Here's how the part is built. I have some questions about the finished solid (model axes, mm). A direction names the side the tool comes from. Round coordinates to 2 decimals unless told otherwise and drop trailing zeros. Loops run counter-clockwise (first coordinate to the right, second up) from the corner with the lowest first, then second, coordinate; pieces in that order, holes last. Notation, with made-up numbers: (44, 52) -> (79, 52) arc R14 cw to (79, 68) -> close; hole circle Ø3 at (43, 56.25). An arc over 180 degrees is marked (long way). One line per item, written item: value. Start each with the question number.
```python
from build123d import *

# Parameters (mm, degrees)
MICRO_SERVO_MOUNT_BASE_PART_CAMERA_TUR_DEPTH = 17.2796
MICRO_START                                  = -8.24
MICRO_SERVO_MOUNT_BASE_PART_CAMERA_3_O_R     = 1.2
MICRO_SERVO_MOUNT_BASE_PART_CAMERA_3_DEPTH   = 16.48
SKETCH7_W                                    = 46
SKETCH7_H                                    = 30
BOSS_EXTRUDE1_DEPTH                          = 3.5
BOSS_EXTRUDE1_DIRECTION_2_REACH              = 35.842
M2_5_CLEARANCE_HOLE1_D                       = 2.9
FILLET1_R                                    = 3
BOSS_EXTRUDE2_DEPTH                          = 10
SKETCH11_R                                   = 2.5
BOSS_EXTRUDE3_DEPTH                          = 8
SKETCH14_W                                   = 17.2796
SKETCH14_H                                   = 27.0711
BOSS_EXTRUDE5_DEPTH                          = 1
BOSS_EXTRUDE4_DEPTH                          = 5
SKETCH13_W                                   = 1.5
SKETCH13_H                                   = 4.25
CUT_EXTRUDE1_DEPTH                           = 39.791353434
FILLET2_R                                    = 2
CUT_EXTRUDE2_DEPTH                           = 2.25
CUT_EXTRUDE3_DEPTH                           = 61.415771958
CHAMFER1_SIZE                                = 0.5


with BuildPart() as part:
    # Micro Servo Mount Base Part - Camera Tur: read off the stored shape, not the designer's step
    # Micro Servo Mount Base Part - Camera 2 → Micro Servo Mount Base Part - Camera Tur (new body)
    with BuildSketch(Plane.YZ):
        Polygon((-23.9811, 0.5), (-16.8311, 0.5), (-16.8311, 6.24), (6.24, 6.24), (6.24, 2.4478), (8.74, 2.4478), (8.74, -2.4478), (6.24, -2.4478), (6.24, -6.24), (-16.8311, -6.24), (-16.8311, -0.5), (-23.9811, -0.5), (-23.9811, -2), (-18.8311, -2), (-18.8311, -8.24), (8.24, -8.24), (8.24, -5), (10.24, -3.5), (10.24, 3.5), (8.24, 5), (8.24, 8.24), (-18.8311, 8.24), (-18.8311, 2), (-23.9811, 2), align=None)
    extrude(amount=MICRO_SERVO_MOUNT_BASE_PART_CAMERA_TUR_DEPTH)

    # Micro Servo Mount Base Part - Camera 3 o → Micro Servo Mount Base Part - Camera 3 (cut)
    with BuildSketch(Plane.XY.offset(MICRO_START)):
        with BuildLine():
            Line((0, -23.9811), (3, -23.9811))
            ThreePointArc((3, -23.9811), (0.878679656, -23.102420344), (0, -20.9811))
            Line((0, -20.9811), (0, -23.9811))
        make_face()
        with BuildLine():
            ThreePointArc((17.2796, -20.9811), (16.400920344, -23.102420344), (14.2796, -23.9811))
            Line((14.2796, -23.9811), (17.2796, -23.9811))
            Line((17.2796, -23.9811), (17.2796, -20.9811))
        make_face()
        with Locations((3, -20.9811)):
            Circle(MICRO_SERVO_MOUNT_BASE_PART_CAMERA_3_O_R)
        with Locations((14.2796, -20.9811)):
            Circle(MICRO_SERVO_MOUNT_BASE_PART_CAMERA_3_O_R)
    extrude(amount=MICRO_SERVO_MOUNT_BASE_PART_CAMERA_3_DEPTH, mode=Mode.SUBTRACT)

    # Sketch7 → Boss-Extrude1 (add)
    with BuildSketch(Plane.XY.offset(8.24)):
        with Locations((13.6398, 0)):
            Rectangle(SKETCH7_W, SKETCH7_H)
    extrude(amount=BOSS_EXTRUDE1_DEPTH)

    # Boss-Extrude1 direction 2: up to this face of the body (flat: up to its plane)
    boss_extrude1_direction_2_end = Plane(part.part.faces().sort_by_distance((8.6398, -5.29555, 6.24))[0])
    # Sketch7 → Boss-Extrude1 direction 2 (add, up to the picked face)
    with BuildSketch(Plane.XY.offset(8.24), mode=Mode.PRIVATE) as boss_extrude1_direction_2_sk1:
        with Locations((13.6398, 0)):
            Rectangle(SKETCH7_W, SKETCH7_H)
    boss_extrude1_direction_2_tool1 = split(extrude(boss_extrude1_direction_2_sk1.sketch, amount=-BOSS_EXTRUDE1_DIRECTION_2_REACH, mode=Mode.PRIVATE), bisect_by=boss_extrude1_direction_2_end, keep=Keep.BOTH, mode=Mode.PRIVATE)
    add(boss_extrude1_direction_2_tool1.solids().sort_by(Axis((13.6398, 0, 8.24), (0, 0, -1)))[0])

    # M2.5 Clearance Hole1 (through all)
    with Locations(Plane.XY.offset(11.74)):
        with Locations((-6.3602, 12), (33.6398, 12), (33.6398, -12), (-6.3602, -12)):
            Hole(M2_5_CLEARANCE_HOLE1_D / 2)

    # Fillet1
    fillet1_edges = [part.edges().sort_by_distance(p)[0] for p in [
        (36.6398, -15, 8.99),
        (-9.3602, 15, 8.99),
        (-9.3602, -15, 8.99),
        (36.6398, 15, 8.99),
    ]]
    fillet(fillet1_edges, radius=FILLET1_R)

    # Sketch10 → Boss-Extrude2 (add)
    with BuildSketch(Plane(origin=(36.6398, 0, 0), x_dir=(0, 0, -1), z_dir=(1, 0, 0))):
        with BuildLine():
            Line((-6.24, 3.5), (0, 3.5))
            ThreePointArc((0, 3.5), (3.5, 0), (0, -3.5))
            Line((0, -3.5), (-6.24, -3.5))
            Line((-6.24, -3.5), (-6.24, 3.5))
        make_face()
    extrude(amount=-BOSS_EXTRUDE2_DEPTH)

    # Sketch11 → Boss-Extrude3 (add)
    with BuildSketch(Plane(origin=(36.6398, 0, 0), x_dir=(0, 0, -1), z_dir=(1, 0, 0))):
        Circle(SKETCH11_R)
    extrude(amount=BOSS_EXTRUDE3_DEPTH)

    # Sketch14 → Boss-Extrude5 (add)
    with BuildSketch(Plane(origin=(0, 0, -8.24), x_dir=(-1, 0, 0), z_dir=(0, 0, -1))):
        with Locations((-8.6398, -5.29555)):
            Rectangle(SKETCH14_W, SKETCH14_H)
    extrude(amount=BOSS_EXTRUDE5_DEPTH)

    # Sketch12 → Boss-Extrude4 (add, symmetric)
    with BuildSketch(Plane(origin=(0, -6.87055, 0), x_dir=(1, 0, 0), z_dir=(0, 1, 0))):
        Polygon((0, 9.74), (0.5148, 9.74), (0.5148, 9.24), (0, 9.24), (0, 6.24), (-1.5, 6.24), (-1.5, 9.74), align=None)
        Polygon((17.2796, 6.24), (18.7796, 6.24), (18.7796, 9.74), (17.2796, 9.74), (16.7648, 9.74), (16.7648, 9.24), (17.2796, 9.24), align=None)
    extrude(amount=BOSS_EXTRUDE4_DEPTH, both=True)

    # Sketch13 → Cut-Extrude1 (cut, through all)
    with BuildSketch(Plane(origin=(18.7796, 0, 0), x_dir=(0, 0, -1), z_dir=(1, 0, 0))):
        with Locations((6.99, -6.87055)):
            Rectangle(SKETCH13_W, SKETCH13_H)
    extrude(amount=-CUT_EXTRUDE1_DEPTH, mode=Mode.SUBTRACT)

    # Fillet2
    fillet2_edges = [part.edges().sort_by_distance(p)[0] for p in [
        (8.6398, -18.8311, -9.24),
        (8.6398, 8.24, -9.24),
    ]]
    fillet(fillet2_edges, radius=FILLET2_R)

    # Sketch15 → Cut-Extrude2 (cut)
    with BuildSketch(Plane(origin=(0, 0, 6.24), x_dir=(-1, 0, 0), z_dir=(0, 0, -1))):
        Polygon((9.3602, 13.732050808), (6.3602, 15.464101615), (3.3602, 13.732050808), (3.3602, 10.267949192), (6.3602, 8.535898385), (9.3602, 10.267949192), align=None)
        Polygon((9.3602, -10.267949192), (6.3602, -8.535898385), (3.3602, -10.267949192), (3.3602, -13.732050808), (6.3602, -15.464101615), (9.3602, -13.732050808), align=None)
        Polygon((-36.6398, -10.267949192), (-36.6398, -13.732050808), (-33.6398, -15.464101615), (-30.6398, -13.732050808), (-30.6398, -10.267949192), (-33.6398, -8.535898385), align=None)
        Polygon((-36.6398, 13.732050808), (-36.6398, 10.267949192), (-33.6398, 8.535898385), (-30.6398, 10.267949192), (-30.6398, 13.732050808), (-33.6398, 15.464101615), align=None)
    extrude(amount=-CUT_EXTRUDE2_DEPTH, mode=Mode.SUBTRACT)

    # Sketch16 → Cut-Extrude3 (cut, through all)
    with BuildSketch(Plane(origin=(0, 15, 0), x_dir=(1, 0, 0), z_dir=(0, 1, 0))):
        Polygon((2.6398, -11.74), (6.1398, -8.24), (21.1398, -8.24), (24.6398, -11.74), align=None)
    extrude(amount=-CUT_EXTRUDE3_DEPTH, mode=Mode.SUBTRACT)

    # Chamfer1
    chamfer1_edges = [part.edges().sort_by_distance(p)[0] for p in [
        (35.1398, 9.401923789, 6.24),
        (32.1398, 9.401923789, 6.24),
        (30.6398, 12, 6.24),
        (31.737876211, 14.366025404, 6.24),
        (31.737876211, -14.366025404, 6.24),
        (30.6398, -12, 6.24),
        (32.1398, -9.401923789, 6.24),
        (35.1398, -9.401923789, 6.24),
        (-7.8602, -9.401923789, 6.24),
        (-4.8602, -9.401923789, 6.24),
        (-3.3602, -12, 6.24),
        (-4.458276211, -14.366025404, 6.24),
        (-4.458276211, 14.366025404, 6.24),
        (-3.3602, 12, 6.24),
        (-4.8602, 9.401923789, 6.24),
        (-7.8602, 9.401923789, 6.24),
    ]]
    chamfer(chamfer1_edges, length=CHAMFER1_SIZE)


solid = part.part
```
Q1. I want a section at D-D on y = -18. Please give me the cut outline in (x, z).
Q2. I want a section at A-A on y = 0. Please give me the cut outline in (x, z).
Q3. Will these pins go through, and if not, where does the flat tip stop? P1, Ø1.8, axis at y = -17.5, z = 2.5, coming from the -X side; P2, Ø1, axis at x = -1, z = -8.5, coming from the -Y side; P3, Ø5, axis at x = 6.5, y = -1, coming from the +Z side.
Q4. If I drill on line 1 along X through (y, z) = (-21, 0.75); line 2 along Z through (x, y) = (7, 8.5) (3 decimals); line 3 along Z through (x, y) = (16.5, 1.5), over which ranges is the centre line in solid material (lowest first)?
Q5. Which directions (+Z, -Z, +X, -X, +Y, -Y) give clear straight access to the entire face, cutting with the end or side of a thin tool? Please do faces 1 (the flat face through (32, -3.5, 3)), 2 (the flat face through (9, -20, 0.5)), 3 (the flat face through (35, 13, 8.49)).
Q6. I want a section at B-B on z = 10.5. Please give me the cut outline in (x, y), plus the area to 3 significant figures.
Q7. If we mould it in two halves opening along Z, with no side actions, what happens to faces 4 (the cylindrical face through (40.58, -2.44, 0.54)), 5 (the flat face through (9, -23.981, -1)), 6 (the flat face through (9, -8.996, -7))? For each: released by +Z, released by -Z, zero draft, split by the parting line, or undercut.
Q8. I want a section at C-C on x = 26. Please give me the cut outline in (y, z).
Answers below:
1. outline: (0, -8.86) -> (17.28, -8.86) -> (17.28, -0.5) -> (0, -0.5) -> close; (0, 0.5) -> (17.28, 0.5) -> (17.28, 8.24) -> (0, 8.24) -> close
2. outline: (-9.36, 6.24) -> (26.64, 6.24) -> (26.64, -3.5) -> (36.64, -3.5) -> (36.64, -2.5) -> (44.64, -2.5) -> (44.64, 2.5) -> (36.64, 2.5) -> (36.64, 11.74) -> (24.64, 11.74) -> (21.14, 8.24) -> (6.14, 8.24) -> (2.64, 11.74) -> (-9.36, 11.74) -> close; (0, -9.24) -> (17.28, -9.24) -> (17.28, -6.24) -> (0, -6.24) -> close
3. P1: stops at x = 0
3. P2: stops at y = -11.87
3. P3: stops at z = 10.38
4. line 1: x = 0 to 1.8, 4.2 to 13.08, 15.48 to 17.28
4. line 2: z = -4.805 to -2.448, 2.448 to 4.805, 6.24 to 8.24
4. line 3: z = -9.24 to -6.24, 6.24 to 8.24
5. face 1: -Z, +X, -X, -Y
5. face 2: +X, -X, -Y
5. face 3: -Z
6. outline: (-9.36, -12) arc R3 ccw to (-6.36, -15) -> (3.88, -15) -> (3.88, 15) -> (-6.36, 15) arc R3 ccw to (-9.36, 12) -> close; (23.4, -15) -> (33.64, -15) arc R3 ccw to (36.64, -12) -> (36.64, 12) arc R3 ccw to (33.64, 15) -> (23.4, 15) -> close; hole circle Ø2.9 at (-6.36, -12); hole circle Ø2.9 at (-6.36, 12); hole circle Ø2.9 at (33.64, -12); hole circle Ø2.9 at (33.64, 12)
6. area: 760 mm^2
7. face 4: split by the parting line
7. face 5: zero draft
7. face 6: undercut
8. outline: (-15, 6.24) -> (15, 6.24) -> (15, 11.74) -> (-15, 11.74) -> close
